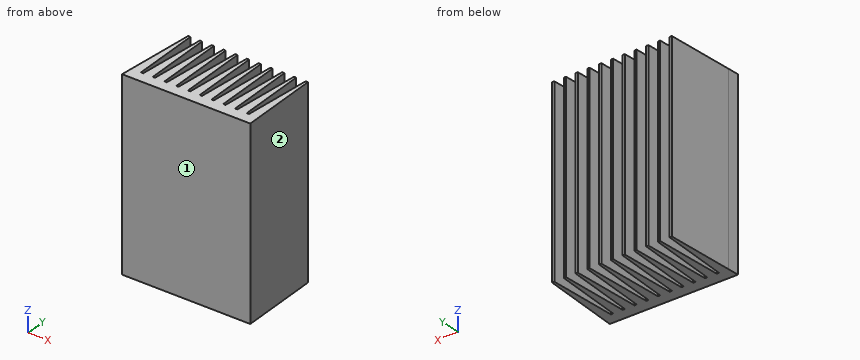
from build123d import *

# Parameters (mm, degrees)
BOSS_EXTRUDE1_DEPTH = 80


with BuildPart() as part:
    # Sketch1 → Boss-Extrude1 (new body)
    with BuildSketch(Plane.XY):
        Polygon((-24.257476664, 0), (0, 0), (13.70186971, 0), (11.867597435, 35), (10.867597435, 35), (9.295364057, 5), (8.295364057, 5), (6.723130678, 35), (5.723130678, 35), (4.1508973, 5), (3.150897297, 5), (1.578663918, 35), (0.578663918, 35), (-0.99356946, 5), (-1.993569463, 5), (-3.565802842, 35), (-4.565802842, 35), (-6.13803622, 5), (-7.138036223, 5), (-8.710269602, 35), (-9.710269602, 35), (-11.28250298, 5), (-12.282502983, 5), (-13.854736362, 35), (-14.854736362, 35), (-16.42696974, 5), (-17.426969743, 5), (-18.999203122, 35), (-19.999203122, 35), (-21.5714365, 5), (-22.571436503, 5), (-24.143669882, 35), (-25.143669882, 35), (-26.71590326, 5), (-27.715903263, 5), (-29.288136642, 35), (-30.288136642, 35), (-31.86037002, 5), (-32.860370023, 5), (-34.432603402, 35), (-35.432603402, 35), (-37.00483678, 5), (-38.004836783, 5), (-39.577070162, 35), (-40.577070162, 35), (-42.14930354, 5), (-42.411342437, 0), align=None)
    extrude(amount=BOSS_EXTRUDE1_DEPTH)


solid = part.part
The listing builds one solid part. Answer for the finished solid, in the listing's coordinates (mm). Face numbers are marked on the shaded views. Give positions to 0.01 mm unless a question says otherwise; leave off trailing zeros. One line per question, with ' | ' between items. Start each with the question number.
1. Section A-A (y = 27) is taken. State how many separate pieces and enclosed holes the cut face has, plus the area to 3 significant figures.
2. Given pin 1 Ø0.5 at (x, z) = (-6.5, 44) entering from +Y; pin 2 Ø8 at (y, z) = (6, 42.5) entering from +X; pin 3 Ø10 at (y, z) = (20.5, 62) entering from -X, each flat-ended and moving along its own axis, determine where each tip first touches the part or whether it passes through.
3. For a pull along X with two mould halves and no side action, classify the marked faces 1 and 2 as pulls with the +X half, pulls with the -X half, needs draft (parallel to the pull), parting line crosses it, or undercut.
4. Find the intervals of material crossed by probe 1 along Y at (x, z) = (-32, 54); probe 2 along X at (y, z) = (3.5, 44.5), in increasing order.
Response values:
1) separate pieces: 11 | enclosed holes: 0 | area: 1,620 mm2
2) pin 1: y = 5 | pin 2: x = 13.6 | pin 3: x = -41.6
3) face 1: needs draft | face 2: pulls with the +X half
4) probe 1: 0 to 5 | probe 2: -42.23 to 13.52
